from build123d import *

# Parameters (mm, degrees)
F0_W     = 1219.2
F0_H     = 609.6
F1_DEPTH = 304.8
F1_TAPER = 3.5
F3_DEPTH = 1219.201
F5_DEPTH = 609.601


with BuildPart() as f1:
    # F0 (on Top) → F1 (new body)
    with BuildSketch(Plane.XY):
        with Locations((609.6, 304.8)):
            Rectangle(F0_W, F0_H)
    extrude(amount=F1_DEPTH, taper=F1_TAPER)

    # F2 (on Right) → F3 (cut, through all)
    with BuildSketch(Plane.YZ):
        Polygon((18.6423666219, 304.8), (0, 9.525), (38.1758597789, 9.525), (56.8182264007, 304.8), align=None)
        Polygon((570.8415662642, 9.525), (609.0174260431, 9.525), (590.9576333781, 304.8), (552.7817735993, 304.8), align=None)
    extrude(amount=F3_DEPTH, mode=Mode.SUBTRACT)

    # F4 (on Front) → F5 (cut, through all)
    with BuildSketch(Plane.XZ):
        Polygon((18.6423666219, 304.8), (0.5825739569, 9.525), (38.7537709338, 9.525), (56.8135635987, 304.8), align=None)
        Polygon((1218.6174260431, 9.525), (1200.5576333781, 304.8), (1162.3864364013, 304.8), (1180.4462290662, 9.525), align=None)
    extrude(amount=-F5_DEPTH, mode=Mode.SUBTRACT)


solid = f1.part
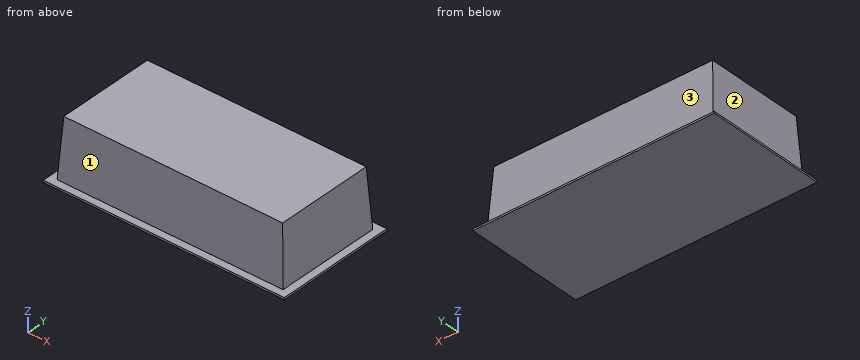
Build history of the part. All positions in model axes, mm. Face numbers are marked on the shaded views. Coordinates: 2 decimals unless noted, no trailing zeros. Write each loop counter-clockwise with the first axis right and the second up, starting at its lowest first coordinate (ties: lowest second). Pieces come first, ordered by that corner, then holes.
(1) Cut at A-A on y = 194. List the corners of the cut face in (x, z) (3 decimals), and give its area (3 significant figures).
(2) Drill centre lines: line 1 (Z direction, x = 609.5, y = 576) (3 decimals); line 2 (Y direction, x = 897, z = 13); line 3 (Y direction, x = 465, z = 53.5). Where is each one in solid material? Low to high.
(3) Cut at D-D on z = 104.5. List the corners of the cut face in (x, y).
(4) Cut at C-C on z = 182. List the corners of the cut face in (x, y).
(5) Mould opens along Y. For the marked faces 1, 2 and 3 say: pulls with the +Y half, pulls with the -Y half, needs draft (parallel to the pull), parting line crosses it, or undercut.
(6) Cut at B-B on x = 281. List the corners of the cut face in (y, z) (3 decimals).
(7) Pin check, flat tips, straight feed: pin 1 Ø10 at (x, y) = (387.5, 227) entering from -Z; pin 2 Ø10 at (y, z) = (433.5, 41) entering from +X; pin 3 Ø1.5 at (x, z) = (360, 114) entering from +Y; pin 4 Ø5 at (x, z) = (390.5, 128.5) entering from -Y. Stop position of each tip, or through.
Working result:
1. outline: (0, 0) - (1219.2, 0) - (1218.617, 9.525) - (1180.446, 9.525) - (1162.386, 304.8) - (56.814, 304.8) - (38.754, 9.525) - (0.583, 9.525) - close
1. area: 343,000 mm2
2. line 1: z = 0 to 9.525
2. line 2: y = 38.4 to 570.63
2. line 3: y = 40.95 to 568.15
3. outline: (44.56, 44.17) - (1174.64, 44.17) - (1174.64, 565.03) - (44.56, 565.03) - close
4. outline: (49.3, 49.07) - (1169.9, 49.07) - (1169.9, 560.29) - (49.3, 560.29) - close
5. face 1: pulls with the -Y half
5. face 2: needs draft
5. face 3: pulls with the +Y half
6. outline: (0, 0) - (609.6, 0) - (609.017, 9.525) - (570.842, 9.525) - (552.782, 304.8) - (56.818, 304.8) - (38.176, 9.525) - (0.583, 9.525) - close
7. pin 1: stops at z = 0
7. pin 2: stops at x = 1178.83
7. pin 3: stops at y = 564.5
7. pin 4: stops at y = 45.53
